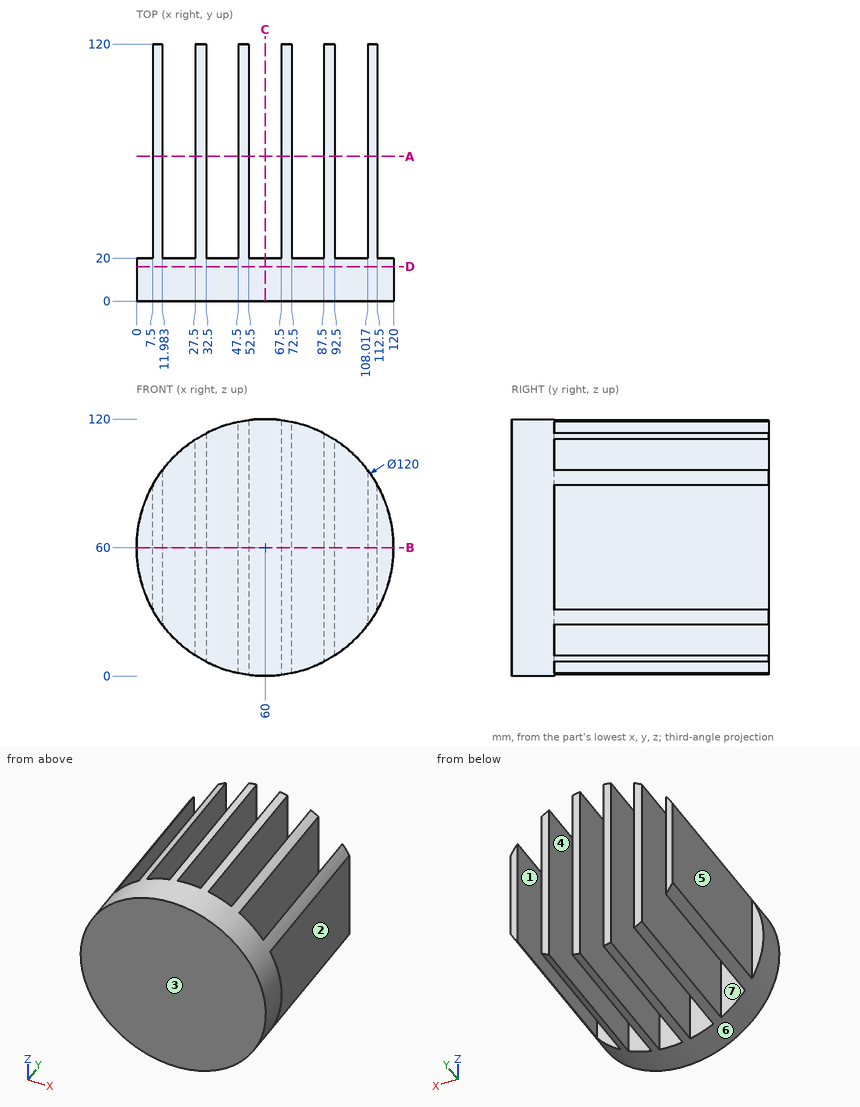
Can you work these out from the drawing? Everything is in mm from the part's minimum corner. A direction names the side the tool comes from. Give positions to 0.01 mm unless a question says otherwise; leave off trailing zeros. Order: outer loops, then holes, each group sorted by start corner. A loop starts at its lowest first (then second) coordinate and runs counter-clockwise, first axis right, second up.
Item 1: I need wall thicknesses on line 1 (X direction, y = 21, z = 43); line 2 (X direction, y = 66, z = 99); line 3 (X direction, y = 33, z = 9). Which ranges of each line are inside material? Lowest first, please.
Item 2: If we section it at B-B, the plane z = 60: Write out the boundary of the cut face in (x, y).
Item 3: If we section it at D-D, the plane y = 16: Write out the boundary of the cut face in (x, z).
Item 4: If we mould it in two halves opening along X, with no side actions, what happens to the marked faces 1, 2, 3 and 4? For each: pulls with the +X half, pulls with the -X half, needs draft (parallel to the pull), parting line crosses it, or undercut.
Item 5: If we section it at C-C, the plane x = 60: Write out the boundary of the cut face in (y, z), plus the area to 3 significant figures.
Item 6: I'm going to push flat-ended pins straight in: pin 1 (4 mm diameter, centred on x = 2.5, z = 48.5, fed in from +Y); pin 2 (10 mm diameter, centred on y = 23.5, z = 79.5, fed in from +X); pin 3 (5 mm diameter, centred on x = 56.5, y = 40.5, fed in from -Z); pin 4 (21.5 mm diameter, centred on y = 63, z = 57, fed in from +X). Where does each tip first touch, or does it pass through?
Item 7: If we section it at A-A, the plane y = 67.5: Write out the boundary of the cut face in (x, z).
Item 8: For the marked faces 5, 6 and 7, which set-ups out of +Z, -Z, +X, -X, +Y, -Y let a thin tool reach every point of the face, with its end or its side?
Values:
1. line 1: x = 7.5 to 11.98, 27.5 to 32.5, 47.5 to 52.5, 67.5 to 72.5, 87.5 to 92.5, 108.02 to 112.5
1. line 2: x = 27.5 to 32.5, 47.5 to 52.5, 67.5 to 72.5, 87.5 to 92.5
1. line 3: x = 28.39 to 32.5, 47.5 to 52.5, 67.5 to 72.5, 87.5 to 91.61
2. outline: (0, 0) - (120, 0) - (120, 20) - (112.5, 20) - (112.5, 120) - (108.02, 120) - (108.02, 20) - (92.5, 20) - (92.5, 120) - (87.5, 120) - (87.5, 20) - (72.5, 20) - (72.5, 120) - (67.5, 120) - (67.5, 20) - (52.5, 20) - (52.5, 120) - (47.5, 120) - (47.5, 20) - (32.5, 20) - (32.5, 120) - (27.5, 120) - (27.5, 20) - (11.98, 20) - (11.98, 120) - (7.5, 120) - (7.5, 20) - (0, 20) - close
3. outline: circle Ø120 at (60, 60)
4. face 1: undercut
4. face 2: pulls with the +X half
4. face 3: needs draft
4. face 4: undercut
5. outline: (0, 0) - (20, 0) - (20, 120) - (0, 120) - close
5. area: 2,400 mm2
6. pin 1: stops at y = 20
6. pin 2: stops at x = 117.85
6. pin 3: passes through
6. pin 4: stops at x = 112.5
7. outline: (7.5, 30.95) arc R60 ccw to (11.98, 24.02) - (11.98, 95.98) arc R60 ccw to (7.5, 89.05) - close; (27.5, 9.56) arc R60 ccw to (32.5, 6.67) - (32.5, 113.33) arc R60 ccw to (27.5, 110.44) - close; (47.5, 1.32) arc R60 ccw to (52.5, 0.47) - (52.5, 119.53) arc R60 ccw to (47.5, 118.68) - close; (67.5, 0.47) arc R60 ccw to (72.5, 1.32) - (72.5, 118.68) arc R60 ccw to (67.5, 119.53) - close; (87.5, 6.67) arc R60 ccw to (92.5, 9.56) - (92.5, 110.44) arc R60 ccw to (87.5, 113.33) - close; (108.02, 24.02) arc R60 ccw to (112.5, 30.95) - (112.5, 89.05) arc R60 ccw to (108.02, 95.98) - close
8. face 5: +Z, -Z, -X, +Y
8. face 6: +Y, -Y
8. face 7: +Z, -Z, +Y
